Verification items for the finished model (mm, model axes). Face numbers are marked on the shaded views. Give positions to 0.01 mm unless a question says otherwise; leave off trailing zeros. Loops run counter-clockwise (first coordinate to the right, second up) from the corner with the lowest first, then second, coordinate; pieces in that order, holes last. Notation, with made-up numbers: (-21, -27.75) -> (-7, -27.75) arc R17 cw to (-7, -14.75) -> close; hole circle Ø8 at (-25, 35.5). An arc over 180 degrees is marked (long way). Answer in a Markdown table with one row per item. Add a question column.
Q1. Material ranges on probe 1 along Y at (x, z) = (0, 8) (3 decimals); probe 2 along Y at (x, z) = (0, 21); probe 3 along X at (y, z) = (-4.5, 10), recorded low to high.
Q2. Gauge pin test, flat ends, axial feed: P1, Ø10, axis at x = 7, z = 10.5, coming from the +Y side; P2, Ø4, axis at x = -3, y = 1.5, coming from the -Z side; P3, Ø1, axis at x = 2.5, y = 8.5, coming from the +Z side. Record the tip position at first contact, or that the pin passes through.
Q3. Section check A-A on z = 19.75. Enter the section's corners in (x, y).
Q4. Section check B-B on z = 26.25. Enter the section's corners in (x, y), and give its area (3 significant figures).
Q5. Release check for a two-part mould opening along X. For the marked faces 1, 2 and 3 record: pulls with the +X half, pulls with the -X half, needs draft (parallel to the pull), parting line crosses it, or undercut.
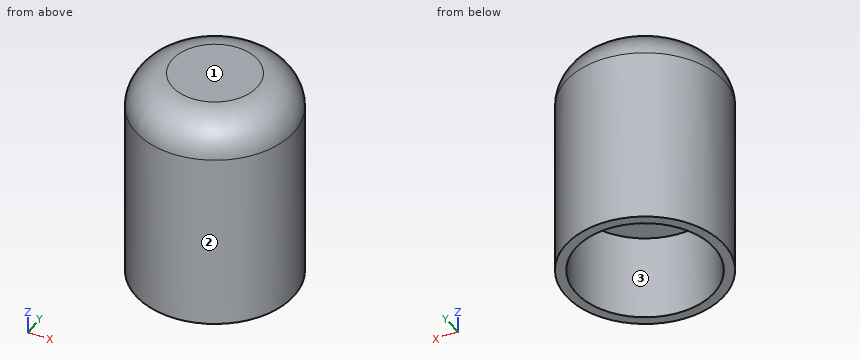
```python
from build123d import *

# Parameters (mm, degrees)
F0_R           = 11
F1_DEPTH       = 30
F2_D           = 10.8
F2_DEPTH       = 25.4
F2_CBORE_D     = 19.25
F2_CBORE_DEPTH = 12
F2_TIP         = 3.2446473427
F3_R           = 5.08


with BuildPart() as f1:
    # F0 (on Top) → F1 (new body)
    with BuildSketch(Plane.XY):
        Circle(F0_R)
    extrude(amount=F1_DEPTH)

    # F2
    with Locations(Plane(origin=(0, 0, 0), x_dir=(1, 0, 0), z_dir=(0, 0, -1))):
        with Locations((0, 0)):
            CounterBoreHole(F2_D / 2, F2_CBORE_D / 2, F2_CBORE_DEPTH, depth=F2_DEPTH)
            with Locations((0, 0, -(F2_DEPTH + F2_TIP / 2))):  # 118° drill point
                Cone(0, F2_D / 2, F2_TIP, mode=Mode.SUBTRACT)

    # F3
    f3_edges = [f1.edges().sort_by_distance(p)[0] for p in [
        (-11, 0, 30),
    ]]
    fillet(f3_edges, radius=F3_R)


solid = f1.part
```
Taken from the geometry:
| question | item | result |
|---|---|---|
| 1 | probe 1 | y = -11 to -9.625, 9.625 to 11 |
| 1 | probe 2 | y = -11 to -5.4, 5.4 to 11 |
| 1 | probe 3 | x = -10.04 to -8.51, 8.51 to 10.04 |
| 2 | P1 | stops at y = 10.82 |
| 2 | P2 | stops at z = 25.43 |
| 2 | P3 | stops at z = 29.38 |
| 3 | outline | circle Ø22 at (0, 0); hole circle Ø10.8 at (0, 0) |
| 4 | outline | circle Ø21.65 at (0, 0); hole circle Ø7.97 at (0, 0) |
| 4 | area | 318 mm² |
| 5 | face 1 | needs draft |
| 5 | face 2 | parting line crosses it |
| 5 | face 3 | undercut |
